from build123d import *

# Parameters (mm, degrees)
CONG_1_R                = 1
ENL_V_MAT_EXTRU_1_REACH = 10.4
ESQUISSE2_R             = 3.25
ESQUISSE2_R_2           = 1.6
ESQUISSE2_R_3           = 1


with BuildPart() as part:
    # Esquisse1 → Révolution1 (revolve)
    with BuildSketch(Plane.XY):
        Polygon((0, 0), (36.071734624, 0), (32.5, -5), (15, -5), (15, -6.4), (5.25, -6.4), (3.25, -8.4), (0, -8.4), align=None)
    revolve(axis=Axis((0, 33.166287016, 0), (0, -1, 0)))

    # Congé1
    cong_1_edges = [part.edges().sort_by_distance(p)[0] for p in [
        (-36.071734624, 0, 0),
    ]]
    fillet(cong_1_edges, radius=CONG_1_R)

    # Esquisse2 → Enlèv. mat.-Extru.1 (cut, up to next)
    with BuildSketch(Plane(origin=(0, 0, 0), x_dir=(1, 0, 0), z_dir=(0, 1, 0)), mode=Mode.PRIVATE) as enl_v_mat_extru_1_sk1:
        Circle(ESQUISSE2_R)
    enl_v_mat_extru_1_tool1 = extrude(enl_v_mat_extru_1_sk1.sketch, amount=-ENL_V_MAT_EXTRU_1_REACH, mode=Mode.PRIVATE) & part.part
    add(enl_v_mat_extru_1_tool1.solids().sort_by_distance((0, 0, 0))[0], mode=Mode.SUBTRACT)
    # Esquisse2 → Enlèv. mat.-Extru.1 (cut, up to next)
    with BuildSketch(Plane(origin=(0, 0, 0), x_dir=(1, 0, 0), z_dir=(0, 1, 0)), mode=Mode.PRIVATE) as enl_v_mat_extru_1_sk2:
        with Locations((10, 0)):
            Circle(ESQUISSE2_R_2)
    enl_v_mat_extru_1_tool2 = extrude(enl_v_mat_extru_1_sk2.sketch, amount=-ENL_V_MAT_EXTRU_1_REACH, mode=Mode.PRIVATE) & part.part
    add(enl_v_mat_extru_1_tool2.solids().sort_by_distance((10, 0, 0))[0], mode=Mode.SUBTRACT)
    # Esquisse2 → Enlèv. mat.-Extru.1 (cut, up to next)
    with BuildSketch(Plane(origin=(0, 0, 0), x_dir=(1, 0, 0), z_dir=(0, 1, 0)), mode=Mode.PRIVATE) as enl_v_mat_extru_1_sk3:
        with Locations((-5, -8.660254038)):
            Circle(ESQUISSE2_R_2)
    enl_v_mat_extru_1_tool3 = extrude(enl_v_mat_extru_1_sk3.sketch, amount=-ENL_V_MAT_EXTRU_1_REACH, mode=Mode.PRIVATE) & part.part
    add(enl_v_mat_extru_1_tool3.solids().sort_by_distance((-5, 0, 8.660254))[0], mode=Mode.SUBTRACT)
    # Esquisse2 → Enlèv. mat.-Extru.1 (cut, up to next)
    with BuildSketch(Plane(origin=(0, 0, 0), x_dir=(1, 0, 0), z_dir=(0, 1, 0)), mode=Mode.PRIVATE) as enl_v_mat_extru_1_sk4:
        with Locations((-5, 8.660254038)):
            Circle(ESQUISSE2_R_2)
    enl_v_mat_extru_1_tool4 = extrude(enl_v_mat_extru_1_sk4.sketch, amount=-ENL_V_MAT_EXTRU_1_REACH, mode=Mode.PRIVATE) & part.part
    add(enl_v_mat_extru_1_tool4.solids().sort_by_distance((-5, 0, -8.660254))[0], mode=Mode.SUBTRACT)
    # Esquisse2 → Enlèv. mat.-Extru.1 (cut, up to next)
    with BuildSketch(Plane(origin=(0, 0, 0), x_dir=(1, 0, 0), z_dir=(0, 1, 0)), mode=Mode.PRIVATE) as enl_v_mat_extru_1_sk5:
        with Locations((-8.5, 14.722431864)):
            Circle(ESQUISSE2_R_3)
    enl_v_mat_extru_1_tool5 = extrude(enl_v_mat_extru_1_sk5.sketch, amount=-ENL_V_MAT_EXTRU_1_REACH, mode=Mode.PRIVATE) & part.part
    add(enl_v_mat_extru_1_tool5.solids().sort_by_distance((-8.5, 0, -14.722432))[0], mode=Mode.SUBTRACT)


solid = part.part
Model file for the job. Use its own axes, mm. A direction names the side the tool comes from. Round coordinates to 2 decimals unless told otherwise and drop trailing zeros. Order: outer loops, then holes, each group sorted by start corner. A loop starts at its lowest first (then second) coordinate and runs counter-clockwise, first axis right, second up.
(1) Pin check, flat tips, straight feed: pin 1 (24 mm diameter, centred on x = -3, z = -2.5, fed in from -Y); pin 2 (2 mm diameter, centred on y = -6.5, z = 6, fed in from +X); pin 3 (3 mm diameter, centred on x = -9, y = -4.5, fed in from +Z); pin 4 (5 mm diameter, centred on y = -4.5, z = 12.5, fed in from -X). Stop position of each tip, or through.
(2) Drill centre lines: line 1 (Y direction, x = 1, z = 8); line 2 (Y direction, x = 21, z = -6); line 3 (X direction, y = -3.75, z = -9). Where is each one in solid material? Low to high.
(3) Band-saw the part on B-B (y = -7.5). List the corners of the cut face in (x, z), then the cut area to 3 significant figures.
(4) 3-axis set-ups, long thin cutter, end or side, ignore diameter. For faces 4 (the face through (-8.63, -2.465, -15.714)), 5 (the face through (14, -5, -7)): which of +Z, -Z, +X, -X, +Y, -Y reach the whole face in a straight line?
(5) Band-saw the part on A-A (z = 0). List the corners of the cut face in (x, y), then the cut area to 3 significant figures.
(6) Band-saw the part on C-C (y = -4). List the corners of the cut face in (x, z).
(7) Pull direction Z, two halves, no side cores. Call faces 1 (the face through (0, 0, -7)), 2 (the face through (31.112, -4.834, 9.798)), 3 (the face through (8.4, -3.16, -0.07)): released by +Z, released by -Z, zero draft, split by the parting line, or undercut.
Verdict:
1. pin 1: stops at y = -8.4
1. pin 2: stops at x = 14.14
1. pin 3: stops at z = 32.78
1. pin 4: stops at x = -32.52
2. line 1: y = -6.4 to 0
2. line 2: y = -5 to 0
2. line 3: x = -32.16 to -6.56, -3.44 to 32.16
3. outline: circle Ø8.3 at (0, 0); hole circle Ø6.5 at (0, 0)
3. area: 20.9 mm2
4. face 4: +Y, -Y
4. face 5: -Y
5. outline: (-34.94, -1.58) - (-32.5, -5) - (-15, -5) - (-15, -6.4) - (-5.25, -6.4) - (-3.25, -8.4) - (-3.25, 0) - (-34.13, 0) arc R1 ccw to start; (3.25, -8.4) - (5.25, -6.4) - (8.4, -6.4) - (8.4, 0) - (3.25, 0) - close; (11.6, -6.4) - (15, -6.4) - (15, -5) - (32.5, -5) - (34.94, -1.58) arc R1 ccw to (34.13, 0) - (11.6, 0) - close
5. area: 325 mm2
6. outline: circle Ø66.43 at (0, 0); hole circle Ø2 at (-8.5, -14.72); hole circle Ø3.2 at (-5, -8.66); hole circle Ø3.2 at (-5, 8.66); hole circle Ø6.5 at (0, 0); hole circle Ø3.2 at (10, 0)
7. face 1: zero draft
7. face 2: split by the parting line
7. face 3: undercut
